from build123d import *

# Parameters (mm, degrees)
SKETCH1_W           = 25.6
SKETCH1_H           = 44.5
BOSS_EXTRUDE1_DEPTH = 15.875
SKETCH2_R           = 3.108453975
SKETCH2_R_2         = 2.615573074
BOSS_EXTRUDE2_DEPTH = 2
FILLET1_R           = 2.54


with BuildPart() as part:
    # Sketch1 → Boss-Extrude1 (new body)
    with BuildSketch(Plane(origin=(0, 0, 0), x_dir=(1, 0, 0), z_dir=(0, 1, 0))):
        with Locations((12.8, 22.25)):
            Rectangle(SKETCH1_W, SKETCH1_H)
    extrude(amount=BOSS_EXTRUDE1_DEPTH)

    # Sketch2 → Boss-Extrude2 (add)
    # profile 1 of 2: a face of its own
    with BuildSketch(Plane(origin=(0, 0, -44.5), x_dir=(-1, 0, 0), z_dir=(0, 0, -1))):
        with Locations(Location((-6.0691761, 7.9375, 0), (0, 0, 180))):
            Circle(SKETCH2_R)
        with Locations((-6.0691761, 7.9375)):
            Circle(SKETCH2_R_2, mode=Mode.SUBTRACT)
    # profile 2 of 2: a face of its own
    with BuildSketch(Plane(origin=(0, 0, -44.5), x_dir=(-1, 0, 0), z_dir=(0, 0, -1))):
        Polygon((-19.490234753, 3.127434709), (-14.490131947, 4.087133188), (-12.821203807, 8.897198479), (-16.152378472, 12.747565291), (-21.152481278, 11.787866812), (-22.821409419, 6.977801521), align=None)
        Polygon((-19.252657716, 3.767035883), (-14.925254294, 4.612681525), (-13.493903191, 8.783145641), (-16.38995551, 12.107964117), (-20.717358932, 11.262318475), (-22.148710035, 7.091854359), align=None, mode=Mode.SUBTRACT)
    extrude(amount=BOSS_EXTRUDE2_DEPTH)

    # Fillet1
    fillet1_edges = [part.edges().sort_by_distance(p)[0] for p in [
        (25.6, 15.875, -22.25),
        (0, 15.875, -22.25),
        (25.6, 0, -22.25),
        (0, 0, -22.25),
    ]]
    fillet(fillet1_edges, radius=FILLET1_R)


solid = part.part
Read the model definition and answer for the solid it produces. Units are mm, in the model's axes. A direction names the side the tool comes from. Round coordinates to 2 decimals unless told otherwise and drop trailing zeros. Write each loop counter-clockwise with the first axis right and the second up, starting at its lowest first coordinate (ties: lowest second). Pieces come first, ordered by that corner, then holes. Notation, with made-up numbers: (-31, 87) - (15, 87) arc R25 ccw to (15, 101) - close; hole circle Ø6 at (-24, 56). An arc over 180 degrees is marked (long way). Use a Markdown table: item, result.
(1) The part is cut by section A-A (x = 7). Write down the section's boundary in (y, z) (3 decimals), then the cut area to 3 significant figures.
Reported:
| item | result |
|---|---|
| outline | (0, -44.5) - (4.972, -44.5) - (4.972, -46.5) - (5.493, -46.5) - (5.493, -44.5) - (10.382, -44.5) - (10.382, -46.5) - (10.903, -46.5) - (10.903, -44.5) - (15.875, -44.5) - (15.875, 0) - (0, 0) - close |
| area | 709 mm2 |
(2) The mould has two halves that part along Y. Classify faces 5 (the flat face through (14.9, 10.4, -45.5)), 6 (the flat face through (14.463, 10.795, -45.486)), 7 (the flat face through (17.03, 3.6, -45.49)): released by +Y, released by -Y, zero draft, split by the parting line, or undercut.
Reported:
| item | result |
|---|---|
| face 5 | undercut |
| face 6 | released by +Y |
| face 7 | released by -Y |
(3) Straight lines are drawn through the part: line 1 along Z through (x, y) = (2.5, 7.5); line 2 along X through (y, z) = (1.25, -32.5); line 3 along Y through (x, z) = (2, -10.5). For each, find the intervals that lie inside material, in ascending order. Write a range as [from, to].
Reported:
| item | result |
|---|---|
| line 1 | [-44.5, 0] |
| line 2 | [0.35, 25.25] |
| line 3 | [0.06, 15.82] |
(4) Each of these flat-tipped pins is pushed along its axis until it touches: pin 1 Ø9 at (x, y) = (19, 7.5) entering from -Z; pin 2 Ø3 at (x, y) = (6.07, 7.94) entering from -Z. Where does it stop, or does it pass through?
Reported:
| item | result |
|---|---|
| pin 1 | z = -46.5 |
| pin 2 | z = -44.5 |
(5) Which of the six approach directions +Z, -Z, +X, -X, +Y, -Y give full straight-line access (tool end or side, diameter ignored) to faces 1 (the flat face through (0, 8, -22)), 2 (the flat face through (13.667, 6.458, -45.486)), 3 (the flat face through (18.617, 12.274, -45.486)), 4 (the flat face through (21.42, 9.21, -45.49))?
Reported:
| item | result |
|---|---|
| face 1 | +Z, -Z, -X, +Y, -Y |
| face 2 | -Z, -Y |
| face 3 | -Z, +X, +Y |
| face 4 | -Z |
(6) The part is cut by section D-D (x = 2). Write down the section's boundary in (y, z).
Reported:
| item | result |
|---|---|
| outline | (0.06, -44.5) - (15.82, -44.5) - (15.82, 0) - (0.06, 0) - close |
(7) The part is cut by section B-B (y = 6). Write down the section's boundary in (x, z).
Reported:
| item | result |
|---|---|
| outline | (0, -44.5) - (3.64, -44.5) - (3.64, -46.5) - (4.31, -46.5) - (4.31, -44.5) - (7.83, -44.5) - (7.83, -46.5) - (8.5, -46.5) - (8.5, -44.5) - (13.83, -44.5) - (13.83, -46.5) - (14.45, -46.5) - (14.45, -44.5) - (21.2, -44.5) - (21.2, -46.5) - (21.98, -46.5) - (21.98, -44.5) - (25.6, -44.5) - (25.6, 0) - (0, 0) - close |
(8) The part is cut by section C-C (y = 2). Write down the section's boundary in (x, z).
Reported:
| item | result |
|---|---|
| outline | (0.06, -44.5) - (25.54, -44.5) - (25.54, 0) - (0.06, 0) - close |
